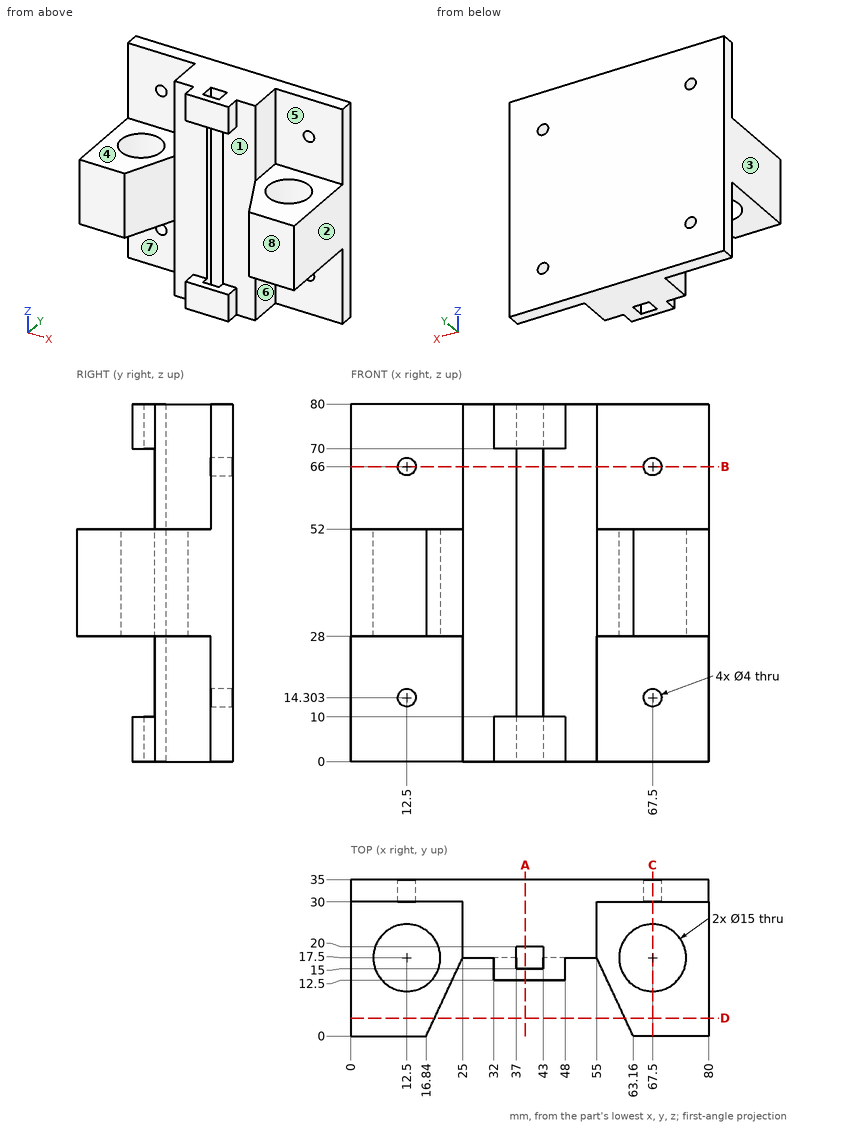
Answer from the drawing. Dimensions are ordinates in mm from the lowest x, y and z of the part. A direction names the side the tool comes from. Give positions to 0.01 mm unless a question says otherwise; leave off trailing zeros. Write each loop counter-clockwise with the first axis right and the second up, starting at its lowest first coordinate (ties: lowest second). Pieces come first, ordered by that corner, then holes.
1) Section B-B (z = 66) is taken. Write down the section's boundary in (x, y).
2) A tool of negligible diameter and unlimited length cuts with its end or side. For the marked faces 4, 5, 6, 7 and 8, from which of +Z, -Z, +X, -X, +Y, -Y can it reach the whole face along a straight path? Write none if from no direction.
3) Find the intervals of material crossed by L1, parallel to X at y = 31.5, z = 66; L2, parallel to Z at x = 67.5, y = 33.45; L3, parallel to Y at x = 67.5, z = 39, in increasing order.
4) Section A-A (x = 39) is taken. Write down the section's boundary in (y, z), and give its area (3 significant figures).
5) Section C-C (x = 67.5) is taken. Write down the section's boundary in (y, z), and give its area (3 significant figures).
6) For a pull along X with two mould halves and no side action, classify the marked faces 1, 2 and 3 as pulls with the +X half, pulls with the -X half, needs draft (parallel to the pull), parting line crosses it, or undercut.
7) Given P1, Ø3, axis at y = 27, z = 24, coming from the +X side; P2, Ø5.5, axis at y = 16, z = 3, coming from the -X side; P3, Ø1, axis at x = 18.5, z = 45.5, coming from the -Y side, each flat-ended and moving along its own axis, determine where each tip first touches the part or whether it passes through.
8) Section D-D (y = 4) is taken. Write down the section's boundary in (x, z) (1 decimal).
Response:
1. outline: (0, 30) - (10.5, 30) - (10.5, 35) - (0, 35) - close; (14.5, 30) - (25, 30) - (25, 17.5) - (37, 17.5) - (37, 20) - (43, 20) - (43, 17.5) - (55, 17.5) - (55, 30) - (65.5, 30) - (65.5, 35) - (14.5, 35) - close; (69.5, 30) - (80, 30) - (80, 35) - (69.5, 35) - close
2. face 4: +Z, -X, -Y
2. face 5: +Z, +X, -Y
2. face 6: -Z, +X, -Y
2. face 7: -Z, -X, -Y
2. face 8: +Z, -Z, +X, -X, -Y
3. L1: x = 0 to 10.5, 14.5 to 65.5, 69.5 to 80
3. L2: z = 0 to 12.3, 16.3 to 64, 68 to 80
3. L3: y = 0 to 10, 25 to 35
4. outline: (12.5, 0) - (15, 0) - (15, 10) - (12.5, 10) - close; (12.5, 70) - (15, 70) - (15, 80) - (12.5, 80) - close; (20, 0) - (35, 0) - (35, 80) - (20, 80) - close
4. area: 1,250 mm2
5. outline: (0, 28) - (10, 28) - (10, 52) - (0, 52) - close; (25, 28) - (30, 28) - (30, 16.3) - (35, 16.3) - (35, 64) - (30, 64) - (30, 52) - (25, 52) - close; (30, 0) - (35, 0) - (35, 12.3) - (30, 12.3) - close; (30, 68) - (35, 68) - (35, 80) - (30, 80) - close
5. area: 720 mm2
6. face 1: undercut
6. face 2: pulls with the +X half
6. face 3: pulls with the -X half
7. P1: stops at x = 55
7. P2: stops at x = 25
7. P3: stops at y = 2.49
8. outline: (0, 28) - (18.7, 28) - (18.7, 52) - (0, 52) - close; (61.3, 28) - (80, 28) - (80, 52) - (61.3, 52) - close
